Could you check a few things on this model? Use its own coordinates, in mm. A direction names the side the tool comes from. Coordinates: 2 decimals unless noted, no trailing zeros. Order: outer loops, then holes, each group sorted by start corner. A loop starts at its lowest first (then second) coordinate and runs counter-clockwise, first axis right, second up. Notation, with made-up numbers: (-14.75, 47.25) - (-6.75, 47.25) arc R13 ccw to (-6.75, 64.25) - close; hole circle Ø11 at (-33.75, -26). An arc over 180 degrees is marked (long way). One line per item, written item: value. Start each with the question number.
from build123d import *

# Parameters (mm, degrees)
MODEL_R                 = 2
MODEL_R_2               = 4.5
MODEL_R_3               = 0.5
MODEL_W                 = 10
MODEL_H                 = 3
SALIENTE_EXTRUIR1_DEPTH = 3


with BuildPart() as part:
    # Model → Saliente-Extruir1 (new body)
    with BuildSketch(Plane.XY):
        with BuildLine():
            Line((0.468281908, 11.04000444), (0.468281908, -14.359995173))
            ThreePointArc((0.468281908, -14.359995173), (1.932748002, -17.895529078), (5.468281908, -19.359995173))
            Line((5.468281908, -19.359995173), (77.465215563, -19.35999556))
            ThreePointArc((77.465215563, -19.35999556), (81.000749469, -17.895529466), (82.465215563, -14.35999556))
            Line((82.465215563, -14.35999556), (82.465215563, -9.05498571))
            Line((82.465215563, -9.05498571), (82.465215563, 11.04000444))
            Line((82.465215563, 11.04000444), (70.665215563, 11.04000444))
            Line((70.665215563, 11.04000444), (70.665215563, 34.24000444))
            Line((70.665215563, 34.24000444), (82.465215563, 34.24000444))
            Line((82.465215563, 34.24000444), (82.465215563, 53.145358109))
            Line((82.465215563, 53.145358109), (82.462149219, 64.823793593))
            Line((82.462149219, 64.823793593), (74.462149219, 64.823793593))
            Line((74.462149219, 64.823793593), (74.462149219, 67.823793593))
            Line((74.462149219, 67.823793593), (82.462149219, 67.823793593))
            Line((82.462149219, 67.823793593), (82.465215563, 72.823793593))
            ThreePointArc((82.465215563, 72.823793593), (81.000749469, 76.359327499), (77.465215563, 77.823793593))
            Line((77.465215563, 77.823793593), (67.948183059, 77.823793593))
            Line((67.948183059, 77.823793593), (45.205743308, 77.823793593))
            Line((45.205743308, 77.823793593), (23.093632519, 77.823793593))
            Line((23.093632519, 77.823793593), (11.942122032, 77.823793593))
            Line((11.942122032, 77.823793593), (5.468281908, 77.823793593))
            ThreePointArc((5.468281908, 77.823793593), (1.932748002, 76.359327499), (0.468281908, 72.823793593))
            Line((0.468281908, 72.823793593), (0.468281908, 67.823793593))
            Line((0.468281908, 67.823793593), (8.468281908, 67.823793593))
            Line((8.468281908, 67.823793593), (8.468281908, 64.823793593))
            Line((8.468281908, 64.823793593), (0.468281908, 64.823793593))
            Line((0.468281908, 64.823793593), (0.468281908, 34.24000444))
            Line((0.468281908, 34.24000444), (12.268281908, 34.24000444))
            Line((12.268281908, 34.24000444), (12.268281908, 11.04000444))
            Line((12.268281908, 11.04000444), (0.468281908, 11.04000444))
        make_face()
        with Locations((55.465215563, 62.823793593)):
            Circle(MODEL_R, mode=Mode.SUBTRACT)
        with Locations((27.465215563, 62.823793593)):
            Circle(MODEL_R, mode=Mode.SUBTRACT)
        with Locations((55.465215563, -14.35999556)):
            Circle(MODEL_R, mode=Mode.SUBTRACT)
        with Locations((27.465215563, -14.35999556)):
            Circle(MODEL_R, mode=Mode.SUBTRACT)
        with Locations((74.565215563, -11.35999556)):
            Circle(MODEL_R_2, mode=Mode.SUBTRACT)
        with Locations((8.365215563, -11.35999556)):
            Circle(MODEL_R_2, mode=Mode.SUBTRACT)
        with Locations((6.365215563, 8.34000444)):
            Circle(MODEL_R_3, mode=Mode.SUBTRACT)
        with Locations((6.365215563, 36.94000444)):
            Circle(MODEL_R_3, mode=Mode.SUBTRACT)
        with Locations((76.565215563, 8.34000444)):
            Circle(MODEL_R_3, mode=Mode.SUBTRACT)
        with Locations((76.565215563, 36.94000444)):
            Circle(MODEL_R_3, mode=Mode.SUBTRACT)
        with Locations((55.465215563, 71.323793593)):
            Rectangle(MODEL_W, MODEL_H, mode=Mode.SUBTRACT)
        with Locations((27.465215563, 71.323793593)):
            Rectangle(MODEL_W, MODEL_H, mode=Mode.SUBTRACT)
    extrude(amount=SALIENTE_EXTRUIR1_DEPTH)


solid = part.part
Q1. I'm going to push flat-ended pins straight in: pin 1 (1.5 mm diameter, centred on x = 79, z = 2, fed in from +Y); pin 2 (3.5 mm diameter, centred on x = 27.47, y = -14.36, fed in from +Z). Where does each tip first touch, or does it pass through?
Q2. If I drill on L1, parallel to Y at x = 73.5, z = 1.5; L2, parallel to Y at x = 54, z = 1.8; L3, parallel to X at y = -10, z = 1.35, over which ranges is the centre line in solid material (lowest first)?
Q3. I want a section at B-B on y = -8. Please give me the cut outline in (x, z), then the cut area to 3 significant figures.
Q4. I want a section at C-C on y = 16. Please give me the cut outline in (x, z).
Q5. We'd pull the mould along X, two halves only. Please class faces 1 (the flat face through (0.468, -1, 1)), 2 (the flat face through (41, 30, 0)), 3 (the flat face through (32.465, 71, 1)): +X half, -X half, draft (parallel to the pull), parting line (faces both ways), or undercut.
Q6. I want a section at D-D on z = 0.8. State how many separate pieces and enclosed holes the cut face has, then the cut area to 3 significant figures.
Q7. I want a section at A-A on x = 59. Please give me the cut outline in (y, z), then the cut area to 3 significant figures.
Q8. Which directions (+Z, -Z, +X, -X, +Y, -Y) give clear straight access to the entire face, cutting with the end or side of a thin tool? Please do faces 4 (the flat face through (5, 64.824, 1)), 5 (the flat face through (27, 69.824, 1)), 6 (the cylindrical face through (81.04, 76.32, 1.48)), 7 (the flat face through (42, 77.824, 1)), 8 (the flat face through (77, 11.04, 1)).
Values follow:
1. pin 1: stops at y = 77.76
1. pin 2: passes through
2. L1: y = -19.36 to -15.73, -6.99 to 11.04, 34.24 to 77.82
2. L2: y = -19.36 to -15.72, -13 to 61.46, 64.19 to 69.82, 72.82 to 77.82
2. L3: x = 0.47 to 4.08, 12.65 to 70.28, 78.85 to 82.47
3. outline: (0.47, 0) - (5.37, 0) - (5.37, 3) - (0.47, 3) - close; (11.36, 0) - (71.57, 0) - (71.57, 3) - (11.36, 3) - close; (77.56, 0) - (82.47, 0) - (82.47, 3) - (77.56, 3) - close
3. area: 210 mm^2
4. outline: (12.27, 0) - (70.67, 0) - (70.67, 3) - (12.27, 3) - close
5. face 1: -X half
5. face 2: draft
5. face 3: undercut
6. separate pieces: 1
6. enclosed holes: 12
6. area: 7,110 mm^2
7. outline: (-19.36, 0) - (69.82, 0) - (69.82, 3) - (-19.36, 3) - close; (72.82, 0) - (77.82, 0) - (77.82, 3) - (72.82, 3) - close
7. area: 283 mm^2
8. face 4: +Z, -Z, -X
8. face 5: +Z, -Z
8. face 6: +Z, -Z, +X, +Y
8. face 7: +Z, -Z, +X, -X, +Y
8. face 8: +Z, -Z, +X
